from build123d import *

# Parameters (mm, degrees)
SKETCH1_R               = 85
SKETCH1_R_2             = 55
BOSS_EXTRUDE1_DEPTH     = 1.5
CUT_EXTRUDE1_DEPTH      = 121.245582039
CUT_EXTRUDE1_DEPTH_BACK = 121.245582039
SKETCH2_R               = 8


with BuildPart() as part:
    # Sketch1 → Boss-Extrude1 (new, symmetric)
    with BuildSketch(Plane(origin=(0, 0, 0), x_dir=(1, 0, 0), z_dir=(0, 1, 0))):
        with Locations(Location((0, 0, 0), (0, 0, 270))):
            Circle(SKETCH1_R)
        with Locations(Location((0, 0, 0), (0, 0, 270))):
            Circle(SKETCH1_R_2, mode=Mode.SUBTRACT)
    extrude(amount=BOSS_EXTRUDE1_DEPTH, both=True)

    # Sketch2 → Cut-Extrude1 (cut, two sides: drawn at the far end of the back side and taken through both)
    with BuildSketch(Plane(origin=(0, 1.5, 0), x_dir=(1, 0, 0), z_dir=(0, 1, 0)).offset(-CUT_EXTRUDE1_DEPTH_BACK)):
        with Locations(Location((70, 0, 0), (0, 0, 270))):
            Circle(SKETCH2_R)
        with Locations(Location((35, -60.621778265, 0), (0, 0, 270))):
            Circle(SKETCH2_R)
        with Locations(Location((-35, -60.621778265, 0), (0, 0, 270))):
            Circle(SKETCH2_R)
        with Locations(Location((-70, 0, 0), (0, 0, 270))):
            Circle(SKETCH2_R)
        with Locations(Location((-35, 60.621778265, 0), (0, 0, 270))):
            Circle(SKETCH2_R)
        with Locations(Location((35, 60.621778265, 0), (0, 0, 270))):
            Circle(SKETCH2_R)
    extrude(amount=CUT_EXTRUDE1_DEPTH + CUT_EXTRUDE1_DEPTH_BACK, mode=Mode.SUBTRACT)


solid = part.part
The model under review builds one solid part; all positions refer to its coordinate system, in mm. Give positions to 0.01 mm unless a question says otherwise; leave off trailing zeros. Loops run counter-clockwise (first coordinate to the right, second up) from the corner with the lowest first, then second, coordinate; pieces in that order, holes last. Notation, with made-up numbers: (33.25, -38.5) -> (80.25, -38.5) arc R9 cw to (80.25, -32.5) -> close; hole circle Ø1 at (74.5, 74.5). An arc over 180 degrees is marked (long way). Put each result on its own line as item: value. Start each with the question number.
1. Mouldability with a two-part tool opening along X and no side actions: class faces 1 (the face through (1.2, -1.5, 55.5)), 2 (the face through (-27.068, -0.021, -61.663)), 3 (the face through (-51.721, 0.021, -67.453)) as released by +X, released by -X, zero draft, split by the parting line, or undercut.
2. We need section D-D on z = -65. State the section outline as (x, y) points.
3. Wall thickness on probe 1 along X at (y, z) = (0.8, 0); probe 2 along X at (y, z) = (-0.3, -55.5); probe 3 along Z at (x, y) = (-35, -0.8): over which ranges is each line inside the solid? List them lowest first.
4. We need section A-A on z = 0. State the section outline as (x, y) points.
5. We need section B-B on y = -0.35. State the section outline as (x, z) points.
6. We need section C-C on x = 0. State the section outline as (y, z) points, then the cut area to 3 significant figures.
Determined:
1. face 1: zero draft
1. face 2: undercut
1. face 3: split by the parting line
2. outline: (-54.77, -1.5) -> (-41.7, -1.5) -> (-41.7, 1.5) -> (-54.77, 1.5) -> close; (-28.3, -1.5) -> (28.3, -1.5) -> (28.3, 1.5) -> (-28.3, 1.5) -> close; (41.7, -1.5) -> (54.77, -1.5) -> (54.77, 1.5) -> (41.7, 1.5) -> close
3. probe 1: -85 to -78, -62 to -55, 55 to 62, 78 to 85
3. probe 2: -64.38 to -41.15, -28.85 to 28.85, 41.15 to 64.38
3. probe 3: -77.46 to -68.62, -52.62 to -42.43, 42.43 to 52.62, 68.62 to 77.46
4. outline: (-85, -1.5) -> (-78, -1.5) -> (-78, 1.5) -> (-85, 1.5) -> close; (-62, -1.5) -> (-55, -1.5) -> (-55, 1.5) -> (-62, 1.5) -> close; (55, -1.5) -> (62, -1.5) -> (62, 1.5) -> (55, 1.5) -> close; (78, -1.5) -> (85, -1.5) -> (85, 1.5) -> (78, 1.5) -> close
5. outline: circle Ø170 at (0, 0); hole circle Ø16 at (-70, 0); hole circle Ø110 at (0, 0); hole circle Ø16 at (-35, -60.62); hole circle Ø16 at (-35, 60.62); hole circle Ø16 at (35, -60.62); hole circle Ø16 at (35, 60.62); hole circle Ø16 at (70, 0)
6. outline: (-1.5, -85) -> (1.5, -85) -> (1.5, -55) -> (-1.5, -55) -> close; (-1.5, 55) -> (1.5, 55) -> (1.5, 85) -> (-1.5, 85) -> close
6. area: 180 mm^2
